Build history of the part. All positions in model axes, mm. A direction names the side the tool comes from. Give positions to 0.01 mm unless a question says otherwise; leave off trailing zeros. Order: outer loops, then holes, each group sorted by start corner. A loop starts at its lowest first (then second) coordinate and runs counter-clockwise, first axis right, second up. Notation, with made-up numbers: (4.25, 63.5) - (20.25, 63.5) arc R18 cw to (20.25, 94.5) - close; hole circle Ø2 at (-10, 41.25). An arc over 180 degrees is marked (long way). Answer in a Markdown table with one row per item.
```python
from build123d import *

# Parameters (mm, degrees)
SKETCH1_W           = 101.6
SKETCH1_H           = 101.6
BOSS_EXTRUDE1_DEPTH = 7.9375
BOSS_EXTRUDE2_DEPTH = 9.525
DRAFT2_ANGLE        = 15
DRAFT3_ANGLE        = 15
FILLET3_R           = 6.35
CUT_EXTRUDE1_REACH  = 31.369
SKETCH3_R           = 1.190625
SKETCH4_R           = 2.38125
CUT_EXTRUDE2_DEPTH  = 6.35
SKETCH5_R           = 2.38125
CUT_EXTRUDE3_DEPTH  = 7.9375
CUT_EXTRUDE4_REACH  = 31.369
SKETCH6_R           = 1.190625
CUT_EXTRUDE5_REACH  = 21.844
SKETCH7_R           = 2.38125
SKETCH7_R_2         = 1.190625
FILLET4_R           = 6.35


with BuildPart() as part:
    # Sketch1 → Boss-Extrude1 (new body)
    with BuildSketch(Plane(origin=(0, 0, 0), x_dir=(1, 0, 0), z_dir=(0, 1, 0))):
        with Locations((50.8, 50.8)):
            Rectangle(SKETCH1_W, SKETCH1_H)
    extrude(amount=BOSS_EXTRUDE1_DEPTH)

    # Sketch2 → Boss-Extrude2 (add)
    with BuildSketch(Plane.ZY.offset(-29.36875)):
        Polygon((-31.75, 7.9375), (-69.85, 7.9375), (-58.57875, 33.3375), (-43.02125, 33.3375), align=None)
    boss_extrude2 = extrude(amount=BOSS_EXTRUDE2_DEPTH)

    # Draft2
    draft2_faces = [part.faces().sort_by_distance(p)[0] for p in [
        (19.84375, 18.858999014, -50.8),
    ]]
    draft(draft2_faces, Plane(origin=(19.84375, 33.3375, -58.57875), x_dir=(0, 0, 1), z_dir=(0, 1, 0)), DRAFT2_ANGLE)

    # Mirror2: Boss-Extrude2 across plane
    add(boss_extrude2.mirror(Plane.ZY.offset(-50.8)))

    # Draft3
    draft3_faces = [part.faces().sort_by_distance(p)[0] for p in [
        (81.75625, 18.858999014, -50.8),
    ]]
    draft(draft3_faces, Plane(origin=(81.75625, 33.3375, -58.57875), x_dir=(0, 0, 1), z_dir=(0, 1, 0)), DRAFT3_ANGLE)

    # Fillet3
    fillet3_edges = [part.edges().sort_by_distance(p)[0] for p in [
        (21.203295256, 7.9375, -31.75),
        (24.60625, 33.3375, -43.02125),
        (24.60625, 33.3375, -58.57875),
        (29.36875, 7.9375, -50.8),
        (21.203295256, 7.9375, -69.85),
        (13.037840512, 7.9375, -50.8),
        (76.99375, 33.3375, -43.02125),
        (88.562159488, 7.9375, -50.8),
        (80.396704744, 7.9375, -31.75),
        (80.396704744, 7.9375, -69.85),
        (76.99375, 33.3375, -58.57875),
        (72.23125, 7.9375, -50.8),
    ]]
    fillet(fillet3_edges, radius=FILLET3_R)

    # Cut-Extrude1: up to this face of the body (flat: up to its plane)
    cut_extrude1_end = Plane(part.part.faces().sort_by_distance((84.905739541, 21.583445016, -50.8))[0])
    # Sketch3 → Cut-Extrude1 (cut, up to the picked face)
    with BuildSketch(Plane.ZY.offset(-72.23125), mode=Mode.PRIVATE) as cut_extrude1_sk1:
        with Locations((-57.8, 30.1625)):
            Circle(SKETCH3_R)
    cut_extrude1_tool1 = split(extrude(cut_extrude1_sk1.sketch, amount=-CUT_EXTRUDE1_REACH, mode=Mode.PRIVATE), bisect_by=cut_extrude1_end, keep=Keep.BOTH, mode=Mode.PRIVATE)
    add(cut_extrude1_tool1.solids().sort_by_distance((72.23125, 30.1625, -57.8))[0], mode=Mode.SUBTRACT)
    # Sketch3 → Cut-Extrude1 (cut, up to the picked face)
    with BuildSketch(Plane.ZY.offset(-72.23125), mode=Mode.PRIVATE) as cut_extrude1_sk2:
        with Locations((-43.8, 30.1625)):
            Circle(SKETCH3_R)
    cut_extrude1_tool2 = split(extrude(cut_extrude1_sk2.sketch, amount=-CUT_EXTRUDE1_REACH, mode=Mode.PRIVATE), bisect_by=cut_extrude1_end, keep=Keep.BOTH, mode=Mode.PRIVATE)
    add(cut_extrude1_tool2.solids().sort_by_distance((72.23125, 30.1625, -43.8))[0], mode=Mode.SUBTRACT)
    # Sketch3 → Cut-Extrude1 (cut, up to the picked face)
    with BuildSketch(Plane.ZY.offset(-72.23125), mode=Mode.PRIVATE) as cut_extrude1_sk3:
        with Locations((-50.8, 23.1625)):
            Circle(SKETCH3_R)
    cut_extrude1_tool3 = split(extrude(cut_extrude1_sk3.sketch, amount=-CUT_EXTRUDE1_REACH, mode=Mode.PRIVATE), bisect_by=cut_extrude1_end, keep=Keep.BOTH, mode=Mode.PRIVATE)
    add(cut_extrude1_tool3.solids().sort_by_distance((72.23125, 23.1625, -50.8))[0], mode=Mode.SUBTRACT)

    # Sketch4 → Cut-Extrude2 (cut)
    with BuildSketch(Plane.ZY.offset(-81.75625)):
        with Locations((-43.8, 30.1625)):
            Circle(SKETCH4_R)
        with Locations((-57.8, 30.1625)):
            Circle(SKETCH4_R)
        with Locations((-50.8, 23.1625)):
            Circle(SKETCH4_R)
    extrude(amount=-CUT_EXTRUDE2_DEPTH, mode=Mode.SUBTRACT)

    # Sketch5 → Cut-Extrude3 (cut)
    with BuildSketch(Plane(origin=(0, 7.9375, 0), x_dir=(1, 0, 0), z_dir=(0, 1, 0))):
        with Locations((10.287, 91.313)):
            Circle(SKETCH5_R)
        with Locations((10.287, 10.287)):
            Circle(SKETCH5_R)
        with Locations((91.313, 10.287)):
            Circle(SKETCH5_R)
        with Locations((91.313, 91.313)):
            Circle(SKETCH5_R)
    extrude(amount=-CUT_EXTRUDE3_DEPTH, mode=Mode.SUBTRACT)

    # Cut-Extrude4: up to this face of the body (flat: up to its plane)
    cut_extrude4_end = Plane(part.part.faces().sort_by_distance((16.694260459, 21.583445016, -50.8))[0])
    # Sketch6 → Cut-Extrude4 (cut, up to the picked face)
    with BuildSketch(Plane(origin=(29.36875, 0, 0), x_dir=(0, 0, -1), z_dir=(1, 0, 0)), mode=Mode.PRIVATE) as cut_extrude4_sk1:
        with Locations((43.3, 22.6625)):
            Circle(SKETCH6_R)
    cut_extrude4_tool1 = split(extrude(cut_extrude4_sk1.sketch, amount=-CUT_EXTRUDE4_REACH, mode=Mode.PRIVATE), bisect_by=cut_extrude4_end, keep=Keep.BOTH, mode=Mode.PRIVATE)
    add(cut_extrude4_tool1.solids().sort_by_distance((29.36875, 22.6625, -43.3))[0], mode=Mode.SUBTRACT)
    # Sketch6 → Cut-Extrude4 (cut, up to the picked face)
    with BuildSketch(Plane(origin=(29.36875, 0, 0), x_dir=(0, 0, -1), z_dir=(1, 0, 0)), mode=Mode.PRIVATE) as cut_extrude4_sk2:
        with Locations((58.3, 22.6625)):
            Circle(SKETCH6_R)
    cut_extrude4_tool2 = split(extrude(cut_extrude4_sk2.sketch, amount=-CUT_EXTRUDE4_REACH, mode=Mode.PRIVATE), bisect_by=cut_extrude4_end, keep=Keep.BOTH, mode=Mode.PRIVATE)
    add(cut_extrude4_tool2.solids().sort_by_distance((29.36875, 22.6625, -58.3))[0], mode=Mode.SUBTRACT)

    # Sketch7 → Cut-Extrude5 (cut, up to next)
    with BuildSketch(Plane(origin=(19.84375, 0, 0), x_dir=(0, 0, -1), z_dir=(1, 0, 0)), mode=Mode.PRIVATE) as cut_extrude5_sk1:
        with Locations((58.3, 22.6625)):
            Circle(SKETCH7_R)
        with Locations((58.3, 22.6625)):
            Circle(SKETCH7_R_2, mode=Mode.SUBTRACT)
    cut_extrude5_tool1 = extrude(cut_extrude5_sk1.sketch, amount=-CUT_EXTRUDE5_REACH, mode=Mode.PRIVATE) & part.part
    add(cut_extrude5_tool1.solids().sort_by_distance((19.84375, 22.6625, -55.986102))[0], mode=Mode.SUBTRACT)
    # Sketch7 → Cut-Extrude5 (cut, up to next)
    with BuildSketch(Plane(origin=(19.84375, 0, 0), x_dir=(0, 0, -1), z_dir=(1, 0, 0)), mode=Mode.PRIVATE) as cut_extrude5_sk2:
        with Locations((43.3, 22.6625)):
            Circle(SKETCH7_R)
        with Locations((43.3, 22.6625)):
            Circle(SKETCH7_R_2, mode=Mode.SUBTRACT)
    cut_extrude5_tool2 = extrude(cut_extrude5_sk2.sketch, amount=-CUT_EXTRUDE5_REACH, mode=Mode.PRIVATE) & part.part
    add(cut_extrude5_tool2.solids().sort_by_distance((19.84375, 22.6625, -40.986102))[0], mode=Mode.SUBTRACT)

    # Fillet4
    fillet4_edges = [part.edges().sort_by_distance(p)[0] for p in [
        (0, 3.96875, -101.6),
        (101.6, 3.96875, -101.6),
        (101.6, 3.96875, 0),
        (0, 3.96875, 0),
    ]]
    fillet(fillet4_edges, radius=FILLET4_R)


solid = part.part
```
1. Which spindle directions (+Z, -Z, +X, -X, +Y, -Y) get a long thin tool onto all of the face, cutting with end or side? Do faces 5 (the face through (24.027, 32.283, -43.646)), 6 (the face through (18.46, 20.55, -44.4)), 7 (the face through (81.756, 29, -57)). Say none if no direction does.
Check result:
| item | result |
|---|---|
| face 5 | +Z, +X, -X, +Y |
| face 6 | -X |
| face 7 | +X |
2. Cut at A-A on z = -50.8. Write the cut outline in (x, y).
Check result:
| item | result |
|---|---|
| outline | (0, 0) - (101.6, 0) - (101.6, 7.94) - (93.43, 7.94) arc R6.35 cw to (87.3, 12.64) - (85.12, 20.78) - (81.76, 20.78) - (81.76, 21.97) - (72.23, 21.97) - (72.23, 14.29) arc R6.35 cw to (65.88, 7.94) - (35.72, 7.94) arc R6.35 cw to (29.37, 14.29) - (29.37, 33.34) - (19.84, 33.34) - (14.3, 12.64) arc R6.35 cw to (8.17, 7.94) - (0, 7.94) - close; (72.23, 24.35) - (81.76, 24.35) - (81.76, 25.54) - (83.84, 25.54) - (81.76, 33.34) - (72.23, 33.34) - close |
3. Drop flat-ended pins along their axis: P1, Ø3, axis at x = 10.287, z = -10.287, coming from the -Y side; P2, Ø3, axis at y = 20, z = -52, coming from the +X side; P3, Ø1.5, axis at x = 16, z = -86.5, coming from the -Y side; P4, Ø1.5, axis at x = 17.5, y = 13.5, coming from the -Z side. Give the stop position or say it passes through.
Check result:
| item | result |
|---|---|
| P1 | passes through |
| P2 | stops at x = 85.73 |
| P3 | stops at y = 0 |
| P4 | stops at z = -67.71 |
4. Probe line 1 (Y direction, x = 79, z = -50.8); line 2 (Y direction, x = 57.5, z = -27.5); line 3 (X direction, y = 25.5, z = -40). List the from-to ranges inside material, lowest first.
Check result:
| item | result |
|---|---|
| line 1 | y = 0 to 21.97, 24.35 to 33.34 |
| line 2 | y = 0 to 7.94 |
| line 3 | x = 17.74 to 29.37, 72.23 to 83.86 |
5. Cut at D-D on z = -80.5. Write the cut outline in (x, y), and give its area (3 significant figures).
Check result:
| item | result |
|---|---|
| outline | (0, 0) - (101.6, 0) - (101.6, 7.94) - (0, 7.94) - close |
| area | 806 mm² |
6. Cut at C-C on z = -65. Write the cut outline in (x, y), and give its area (3 significant figures).
Check result:
| item | result |
|---|---|
| outline | (0, 0) - (101.6, 0) - (101.6, 7.94) - (93.43, 7.94) arc R6.35 cw to (87.3, 12.64) - (85.63, 18.87) - (72.23, 18.87) - (72.23, 14.29) arc R6.35 cw to (65.88, 7.94) - (35.72, 7.94) arc R6.35 cw to (29.37, 14.29) - (29.37, 18.87) - (15.97, 18.87) - (14.3, 12.64) arc R6.35 cw to (8.17, 7.94) - (0, 7.94) - close |
| area | 1,160 mm² |
7. Cut at B-B on x = 54.5. Write the cut outline in (y, z).
Check result:
| item | result |
|---|---|
| outline | (0, -101.6) - (7.94, -101.6) - (7.94, 0) - (0, 0) - close |
8. Two-plate mould, pull along X, no slides. Class faces 1 (the face through (77.77, 20.76, -37.44)), 2 (the face through (72.231, 21.8, -50.6)), 3 (the face through (19.844, 22, -57)), 4 (the face through (81.756, 29, -45)): +X half, -X half, draft (parallel to the pull), parting line (faces both ways), or undercut.
Check result:
| item | result |
|---|---|
| face 1 | draft |
| face 2 | undercut |
| face 3 | -X half |
| face 4 | +X half |
